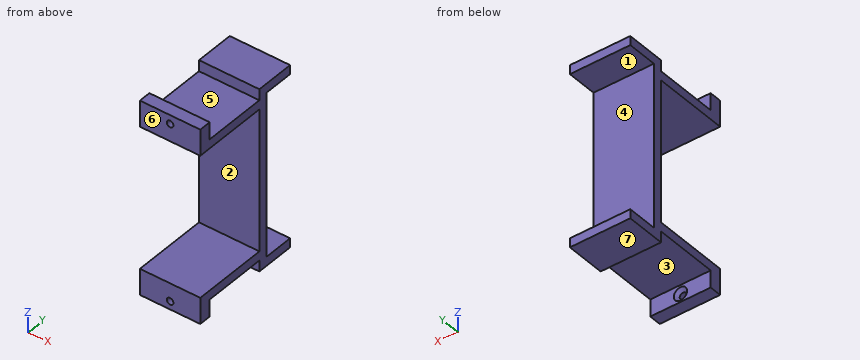
```python
from build123d import *

# Parameters (mm, degrees)
SKETCH1_W                                           = 60.3
SKETCH1_H                                           = 38
BOSS_EXTRUDE1_DEPTH                                 = 10
SKETCH3_W                                           = 20
SKETCH3_H                                           = 54.3
CUT_EXTRUDE1_DEPTH                                  = 10
SKETCH4_W                                           = 20
SKETCH4_H                                           = 47
CUT_EXTRUDE2_DEPTH                                  = 25
SKETCH6_W                                           = 10
SKETCH6_H                                           = 21
CUT_EXTRUDE3_DEPTH                                  = 3.65
SKETCH7_W                                           = 10
SKETCH7_H                                           = 21
CUT_EXTRUDE4_DEPTH                                  = 3.65
MOVE_FACE1_BY                                       = 2
MOVE_FACE1_2_BY                                     = 2
MOVE_FACE2_BY                                       = 10
CSK_FOR_M2_COUNTERSUNK_FLAT_HEAD_SCREW2_D           = 2.2
CSK_FOR_M2_COUNTERSUNK_FLAT_HEAD_SCREW2_DEPTH       = 4
CSK_FOR_M2_COUNTERSUNK_FLAT_HEAD_SCREW2_CSINK_D     = 4.4
CSK_FOR_M2_COUNTERSUNK_FLAT_HEAD_SCREW2_CSINK_ANGLE = 90


with BuildPart() as part:
    # Sketch1 → Boss-Extrude1 (new body)
    with BuildSketch(Plane(origin=(0, 0, 0), x_dir=(0, 0, -1), z_dir=(1, 0, 0))):
        Rectangle(SKETCH1_W, SKETCH1_H)
    extrude(amount=BOSS_EXTRUDE1_DEPTH)

    # Sketch3 → Cut-Extrude1 (cut)
    with BuildSketch(Plane(origin=(0, 19, 0), x_dir=(1, 0, 0), z_dir=(0, 1, 0))):
        Rectangle(SKETCH3_W, SKETCH3_H)
    extrude(amount=-CUT_EXTRUDE1_DEPTH, mode=Mode.SUBTRACT)

    # Sketch4 → Cut-Extrude2 (cut)
    with BuildSketch(Plane.XZ.offset(19)):
        Rectangle(SKETCH4_W, SKETCH4_H)
    extrude(amount=-CUT_EXTRUDE2_DEPTH, mode=Mode.SUBTRACT)

    # Sketch6 → Cut-Extrude3 (cut)
    with BuildSketch(Plane(origin=(0, 0, -30.15), x_dir=(-1, 0, 0), z_dir=(0, 0, -1))):
        with Locations((-5, -4.5)):
            Rectangle(SKETCH6_W, SKETCH6_H)
    extrude(amount=-CUT_EXTRUDE3_DEPTH, mode=Mode.SUBTRACT)

    # Sketch7 → Cut-Extrude4 (cut)
    with BuildSketch(Plane.XY.offset(30.15)):
        with Locations((5, -4.5)):
            Rectangle(SKETCH7_W, SKETCH7_H)
    extrude(amount=-CUT_EXTRUDE4_DEPTH, mode=Mode.SUBTRACT)

    # Move Face1: a face moved outward by 2.0
    extrude(part.faces().sort_by_distance((5, -17, 30.15))[0], amount=MOVE_FACE1_BY, dir=(0, 0, 1))

    # Move Face1 2: a face moved outward by 2.0
    extrude(part.faces().sort_by_distance((5, -17, -30.15))[0], amount=MOVE_FACE1_2_BY, dir=(0, 0, -1))

    # Move Face2: a face moved outward by 10.0
    extrude(part.faces().sort_by_distance((0, 0, 25.72))[0], amount=MOVE_FACE2_BY, dir=(-1, 0, 0))

    # CSK for M2 Countersunk Flat Head Screw2
    with Locations(Plane(origin=(0, -15, 0), x_dir=(1, 0, 0), z_dir=(0, 1, 0))):
        with Locations((0, -29.232676383), (0, 29.454263306)):
            CounterSinkHole(CSK_FOR_M2_COUNTERSUNK_FLAT_HEAD_SCREW2_D / 2, CSK_FOR_M2_COUNTERSUNK_FLAT_HEAD_SCREW2_CSINK_D / 2, depth=CSK_FOR_M2_COUNTERSUNK_FLAT_HEAD_SCREW2_DEPTH, counter_sink_angle=CSK_FOR_M2_COUNTERSUNK_FLAT_HEAD_SCREW2_CSINK_ANGLE)


solid = part.part
```
Model file for the job. Use its own axes, mm. Face numbers are marked on the shaded views. A direction names the side the tool comes from. Coordinates: 2 decimals unless noted, no trailing zeros. Loops run counter-clockwise (first coordinate to the right, second up) from the corner with the lowest first, then second, coordinate; pieces in that order, holes last. Notation, with made-up numbers: (6.25, 87.5) - (20.25, 87.5) arc R23 ccw to (20.25, 113.5) - close; hole circle Ø6 at (36.25, -30.5). An arc over 180 degrees is marked (long way). Write item = value, one per line. Start each with the question number.
Item 1: Saw through at B-B, the plane y = -6. List the corners of the cut face in (x, z).
Item 2: Drop flat-ended pins along their axis: pin 1 Ø8 at (x, z) = (-2.5, -19) entering from +Y; pin 2 Ø8 at (x, y) = (-3.5, 15) entering from -Z; pin 3 Ø2 at (x, y) = (-2.5, -9) entering from -Z. Give the stop position or say it passes through.
Item 3: Saw through at A-A, the plane x = 0. State how many separate pieces and enclosed holes the cut face has, then the cut area to 3 significant figures.
Item 4: Pull direction Z, two halves, no side cores. Call the marked faces 4, 5, 6 and 7: +Z half, -Z half, draft (parallel to the pull), parting line (faces both ways), or undercut.
Item 5: Saw through at D-D, the plane z = -15. List the corners of the cut face in (x, y), then the cut area to 3 significant figures.
Item 6: Saw through at C-C, the plane x = -3.5. List the corners of the cut face in (y, z).
Item 7: 3-axis set-ups, long thin cutter, end or side, ignore diameter. For the marked faces 1, 2 and 3: which of +Z, -Z, +X, -X, +Y, -Y reach the whole face in a straight line?
Item 8: Wall check: probe 1 along Z at (x, y) = (0, -17.7); probe 2 along Z at (x, y) = (-3, 4); probe 3 along Y at (x, z) = (-8.25, 27.5). Give the ranges that are in metal, low to high. Write a range as [from, to].
Answers:
q1.outline = (-10, -26.5) - (10, -26.5) - (10, -23.5) - (-10, -23.5) - close; (-10, 23.5) - (10, 23.5) - (10, 26.5) - (-10, 26.5) - close
q2.pin_1 = 9
q2.pin_2 = -30.15
q2.pin_3 = -26.5
q3.separate_pieces = 3
q3.enclosed_holes = 0
q3.area = 416 mm2
q4.face_4 = undercut
q4.face_5 = +Z half
q4.face_6 = draft
q4.face_7 = -Z half
q5.outline = (-10, 6) - (10, 6) - (10, 9) - (-10, 9) - close
q5.area = 60.0 mm2
q6.outline = (-19, -32.15) - (-15, -32.15) - (-15, -26.5) - (6, -26.5) - (6, -30.15) - (19, -30.15) - (19, -27.15) - (9, -27.15) - (9, 27.15) - (19, 27.15) - (19, 30.15) - (6, 30.15) - (6, 26.5) - (-15, 26.5) - (-15, 32.15) - (-19, 32.15) - (-19, 23.5) - (6, 23.5) - (6, -23.5) - (-19, -23.5) - close
q7.face_1 = +X, -X, +Y
q7.face_2 = +X, -X, -Y
q7.face_3 = -Z, +X, -X
q8.probe_1 = [-32.15, -30.55], [-28.35, -23.5], [23.5, 28.13], [30.33, 32.15]
q8.probe_2 = [-26.5, -23.5], [23.5, 26.5]
q8.probe_3 = [-19, -15], [6, 19]
